Check sheet for the modelled part. Datum: model origin and axes. Units: mm. Face numbers are marked on the shaded views. A direction names the side the tool comes from. Round coordinates to 2 decimals unless told otherwise and drop trailing zeros. Write each loop counter-clockwise with the first axis right and the second up, starting at its lowest first coordinate (ties: lowest second). Pieces come first, ordered by that corner, then holes. Notation, with made-up numbers: (4, 69.25) - (14, 69.25) arc R12 ccw to (14, 92.25) - close; hole circle Ø10 at (-20.5, -26). An arc over 180 degrees is marked (long way). Use one line per item in the form item = value. Start each with the question number.
1) Draft check along X on the marked faces 5, 6 and 7. Enter one of: +X half, -X half, draft (parallel to the pull), parting line (faces both ways), or undercut.
2) Section check D-D (y = 45). Record the boundary of the cut face in (x, z), then the cut area to 3 significant figures.
3) Section check A-A (x = 14). Record the boundary of the cut face in (y, z).
4) Section check B-B (y = 6.5). Record the boundary of the cut face in (x, z).
5) Section check C-C (x = -5.5). Record the boundary of the cut face in (y, z), then the cut area to 3 significant figures.
6) Scan lines: probe 1 along Y at (x, z) = (-14, 0); probe 2 along Y at (x, z) = (12.75, 0); probe 3 along X at (y, z) = (22.5, -6). Record each from-to range of solid material in increasing order.
7) Gauge pin test, flat ends, axial feed: P1, Ø1, axis at x = 6, z = -15.5, coming from the +Y side; P2, Ø8, axis at x = 15, y = 13, coming from the -Z side; P3, Ø7, axis at x = -2.5, y = 15, coming from the +Z side. Record the tip position at first contact, or that the pin passes through.
8) Set-up check for the marked faces 1, 2, 3 and 4: record each of +Z, -Z, +X, -X, +Y, -Y from which the full face is reachable in a straight line by a thin tool's end or side.
from build123d import *

# Parameters (mm, degrees)
SKETCH_1_R          = 10
EXTRUDE_1_DEPTH     = 13
CUT_EXTRUDE_2_DEPTH = 20.209373
SKETCH_7_W          = 30
SKETCH_7_H          = 30
SKETCH_7_R          = 10
EXTRUDE_2_DEPTH     = 8
SKETCH_11_W         = 7
SKETCH_11_H         = 30
EXTRUDE_6_DEPTH     = 50
FILLET_2_R          = 10
SKETCH_13_R         = 8.5
SKETCH_13_R_2       = 7.5
CUT_EXTRUDE_3_DEPTH = 2.5
SKETCH_14_R         = 3.5
CUT_EXTRUDE_4_DEPTH = 37
SKETCH_22_W         = 20
SKETCH_22_H         = 6
EXTRUDE_8_DEPTH     = 18.5
CHAMFER_7_SIZE      = 2
SKETCH_23_R         = 9
CUT_EXTRUDE_6_DEPTH = 3
CHAMFER_8_SIZE      = 2
CUT_EXTRUDE_START   = -5
SKETCH_24_R         = 10
CUT_EXTRUDE_7_DEPTH = 5
CUT_EXTRUDE_START_2 = -2
SKETCH_25_R         = 3
CUT_EXTRUDE_8_DEPTH = 2
CHAMFER_9_SIZE      = 3
CHAMFER_10_SIZE     = 1
CHAMFER_3_SIZE      = 2
EXTRUDE_START       = 5
SKETCH_26_R         = 11.5
SKETCH_26_R_2       = 9
EXTRUDE_9_DEPTH     = 5
CHAMFER_4_SIZE      = 0.5


with BuildPart() as part:
    # 草图1 → 凸台-拉伸1 (new body)
    with BuildSketch(Plane(origin=(0, 0, 0), x_dir=(1, 0, 0), z_dir=(0, 1, 0))):
        with Locations(Location((0, 0, 0), (0, 0, 90))):
            Circle(SKETCH_1_R)
    extrude(amount=EXTRUDE_1_DEPTH)

    # 草图4 → 切除-拉伸2 (cut, through all)
    with BuildSketch(Plane(origin=(0, 13, 0), x_dir=(1, 0, 0), z_dir=(0, 1, 0))):
        with BuildLine():
            Line((3, 0), (-1.5, 2.598076))
            ThreePointArc((-1.5, 2.598076), (-1.5, -2.598076), (3, 0))
        make_face()
    extrude(amount=-CUT_EXTRUDE_2_DEPTH, mode=Mode.SUBTRACT)

    # 草图7 → 凸台-拉伸2 (add)
    with BuildSketch(Plane.XZ):
        Rectangle(SKETCH_7_W, SKETCH_7_H)
        with Locations(Location((0, 0, 0), (0, 0, 270))):
            Circle(SKETCH_7_R, mode=Mode.SUBTRACT)
    extrude(amount=-EXTRUDE_2_DEPTH)

    # 草图11 → 凸台-拉伸6 (add)
    with BuildSketch(Plane.XZ):
        with Locations((-18.5, 0)):
            Rectangle(SKETCH_11_W, SKETCH_11_H)
        with Locations((18.5, 0)):
            Rectangle(SKETCH_11_W, SKETCH_11_H)
    extrude(amount=-EXTRUDE_6_DEPTH)

    # 圆角2
    fillet_2_edges = [part.edges().sort_by_distance(p)[0] for p in [
        (-18.5, 50, -15),
        (-18.5, 50, 15),
        (18.5, 50, 15),
        (18.5, 50, -15),
    ]]
    fillet(fillet_2_edges, radius=FILLET_2_R)

    # 草图13 → 切除-拉伸3 (cut)
    with BuildSketch(Plane(origin=(22, 0, 0), x_dir=(0, 0, -1), z_dir=(1, 0, 0))):
        with Locations((0, 32.5)):
            Circle(SKETCH_13_R)
        with Locations((0, 32.5)):
            Circle(SKETCH_13_R_2, mode=Mode.SUBTRACT)
    cut_extrude_3 = extrude(amount=-CUT_EXTRUDE_3_DEPTH, mode=Mode.SUBTRACT)

    # 草图14 → 切除-拉伸4 (cut)
    with BuildSketch(Plane(origin=(22, 0, 0), x_dir=(0, 0, -1), z_dir=(1, 0, 0))):
        with Locations((0, 32.5)):
            Circle(SKETCH_14_R)
    cut_extrude_4 = extrude(amount=-CUT_EXTRUDE_4_DEPTH, mode=Mode.SUBTRACT)

    # 草图22 → 凸台-拉伸8 (add)
    with BuildSketch(Plane.XZ):
        with Locations((0, -18)):
            Rectangle(SKETCH_22_W, SKETCH_22_H)
    extrude(amount=-EXTRUDE_8_DEPTH)

    # 倒角7
    chamfer_7_edges = [part.edges().sort_by_distance(p)[0] for p in [
        (10, 4, -15),
        (-10, 4, -15),
    ]]
    chamfer(chamfer_7_edges, length=CHAMFER_7_SIZE)

    # 草图23 → 切除-拉伸6 (cut)
    with BuildSketch(Plane.ZY.offset(-15)):
        with Locations((0, 32.5)):
            Circle(SKETCH_23_R)
    cut_extrude_6 = extrude(amount=-CUT_EXTRUDE_6_DEPTH, mode=Mode.SUBTRACT)

    # 倒角8
    chamfer_8_edges = [part.edges().sort_by_distance(p)[0] for p in [
        (10, 18.5, -18),
        (10, 9.25, -21),
        (-10, 18.5, -18),
        (-10, 9.25, -21),
    ]]
    chamfer(chamfer_8_edges, length=CHAMFER_8_SIZE)

    # 草图24 → 切除-拉伸7 (cut)
    with BuildSketch(Plane(origin=(0, 13, 0), x_dir=(1, 0, 0), z_dir=(0, 1, 0)).offset(CUT_EXTRUDE_START)):
        Circle(SKETCH_24_R)
    extrude(amount=CUT_EXTRUDE_7_DEPTH, mode=Mode.SUBTRACT)

    # 草图25 → 切除-拉伸8 (cut)
    with BuildSketch(Plane.XZ.offset(CUT_EXTRUDE_START_2)):
        with Locations(Location((0, 0, 0), (0, 0, 90))):
            Circle(SKETCH_25_R)
    extrude(amount=CUT_EXTRUDE_8_DEPTH, mode=Mode.SUBTRACT)

    # 倒角9
    chamfer_9_edges = [part.edges().sort_by_distance(p)[0] for p in [
        (-22, 0, 0),
        (22, 0, 0),
    ]]
    chamfer(chamfer_9_edges, length=CHAMFER_9_SIZE)

    # 倒角10
    chamfer_10_edges = [part.edges().sort_by_distance(p)[0] for p in [
        (1.5, 0, 2.598076),
    ]]
    chamfer(chamfer_10_edges, length=CHAMFER_10_SIZE)

    # 倒角3
    chamfer_3_edges = [part.edges().sort_by_distance(p)[0] for p in [
        (15, 8, 0),
        (-15, 8, 0),
        (0, 8, -15),
    ]]
    chamfer(chamfer_3_edges, length=CHAMFER_3_SIZE)

    # 草图26 → 凸台-拉伸9 (add)
    with BuildSketch(Plane.ZY.offset(-15).offset(EXTRUDE_START)):
        with Locations((0, 32.5)):
            Circle(SKETCH_26_R)
        with Locations((0, 32.5)):
            Circle(SKETCH_26_R_2, mode=Mode.SUBTRACT)
    extrude_9 = extrude(amount=-EXTRUDE_9_DEPTH)

    # 镜向2: 切除-拉伸3, 切除-拉伸4, 切除-拉伸6, 凸台-拉伸9 across plane
    add(cut_extrude_3.mirror(Plane(origin=(0, 0, 0), x_dir=(0, 0, 1), z_dir=(1, 0, 0))), mode=Mode.SUBTRACT)
    add(cut_extrude_4.mirror(Plane(origin=(0, 0, 0), x_dir=(0, 0, 1), z_dir=(1, 0, 0))), mode=Mode.SUBTRACT)
    add(cut_extrude_6.mirror(Plane(origin=(0, 0, 0), x_dir=(0, 0, 1), z_dir=(1, 0, 0))), mode=Mode.SUBTRACT)
    add(extrude_9.mirror(Plane(origin=(0, 0, 0), x_dir=(0, 0, 1), z_dir=(1, 0, 0))))

    # 倒角4
    chamfer_4_edges = [part.edges().sort_by_distance(p)[0] for p in [
        (10, 32.5, -11.5),
        (-22, 32.5, 3.5),
        (-10, 32.5, -11.5),
        (22, 32.5, 3.5),
    ]]
    chamfer(chamfer_4_edges, length=CHAMFER_4_SIZE)


solid = part.part
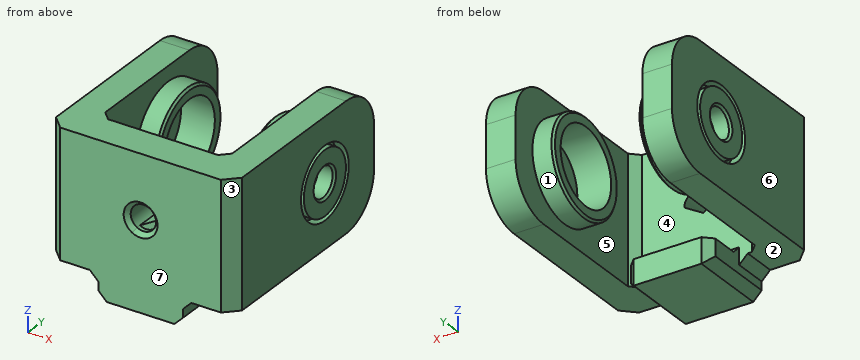
Results are:
q1.face_5 = undercut
q1.face_6 = -X half
q1.face_7 = draft
q2.outline = (-22, -13.66) - (-15, -13.66) - (-15, 13.66) - (-22, 13.66) - close; (15, -13.66) - (22, -13.66) - (22, 13.66) - (15, 13.66) - close
q2.area = 382 mm²
q3.outline = (0, -15) - (9, -15) - (9, 15) - (0, 15) - close; circle Ø23 at (32.5, 0); hole circle Ø18 at (32.5, 0)
q4.outline = (-22, -15) - (-12, -15) - (-10, -17) - (-10, -19) - (-8, -21) - (8, -21) - (10, -19) - (10, -17) - (12, -15) - (22, -15) - (22, 15) - (-22, 15) - close; hole (-1.5, -2.6) - (3, 0) arc R3 ccw (long way) to start
q5.outline = (0, -21) - (18.5, -21) - (18.5, -15) - (10, -15) - (8, -13) - (8, 15) - (0, 15) - close
q5.area = 353 mm²
q6.probe_1 = 0 to 9, 21 to 23.5, 41.5 to 44
q6.probe_2 = 0 to 8, 21 to 23.5, 41.5 to 44
q6.probe_3 = -22 to -15, 15 to 22
q7.P1 = 18.5
q7.P2 = -15
q7.P3 = -15
q8.face_1 = none
q8.face_2 = -Z, -X, +Y, -Y
q8.face_3 = +Z, -Z, +X, -Y
q8.face_4 = +Z
